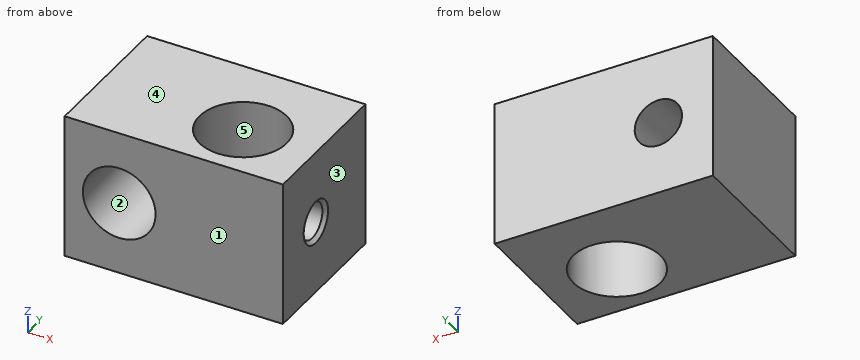
Autodesk Inventor part; units mm, degrees
ref_plane "YZ Plane" through (0, 0, 0) normal (1, 0, 0) x (0, 1, 0)
ref_plane "XZ Plane" through (0, 0, 0) normal (0, 1, 0) x (-1, 0, 0)
ref_plane "XY Plane" through (0, 0, 0) normal (0, 0, 1) x (1, 0, 0)
sketch "Sketch1" plane through (0, 0, 0) normal (0, 0, 1) x (1, 0, 0)
  line L0 (0, 0) -> (30, 0)
  line L1 (30, 0) -> (30, 20)
  line L2 (30, 20) -> (0, 20)
  line L3 (0, 20) -> (0, 0)
  dimension "d0" = 30
  dimension "d1" = 20
extrude "Extrusion1" add sketch "Sketch1" along normal blind 20
sketch "Sketch2" plane through (0, 0, 0) normal (0, -1, 0) x (1, 0, 0)
  line L0 (30, 20) -> (0, 20)
  line L1 (0, 0) -> (0, 20)
  point P0 (7.5, 10)
  dimension "d4" = 7.5
  dimension "d5" = 10
hole "Hole1" at (7.5, 0, 10) direction (0, 1, 0) diameter 6.5 depth 20 tip angle 118 counterbore diameter 10 counterbore depth 13
sketch "Sketch3" plane through (0, 0, 20) normal (0, 0, 1) x (1, 0, 0)
  line L0 (0, 0) -> (0, 20)
  line L1 (0, 20) -> (30, 20)
  point P0 (20, 8)
  dimension "d13" = 20
  dimension "d14" = 12
hole "Hole2" at (20, 8, 20) direction (0, 0, -1) diameter 12 depth 20 tip angle 118
sketch "Sketch4" plane through (30, 0, 0) normal (1, 0, 0) x (0, 0, -1)
  line L0 (0, 0) -> (0, 20)
  line L1 (0, 20) -> (-20, 20)
  point P0 (-10, 8)
  dimension "d22" = 10
  dimension "d23" = 12
hole "Hole3" at (30, 8, 10) direction (-1, 0, 0) diameter 4.917 depth 6 tip angle 118
chamfer "Chamfer1" distance 0.5 angle 45 1 edges at (30, 8, 12.4585)
equation "\"d17\" = d14"
equation "\"d26\" = d14"
properties part number "MANCAL DO EIXO DIANTEIRO(7)" material "Carbon Steel"
Can you work these out from the model? Positions are in its coordinate system, mm. Face numbers are marked on the shaded views. A direction names the side the tool comes from. Coordinates: 2 decimals unless noted, no trailing zeros. Write each loop counter-clockwise with the first axis right and the second up, starting at its lowest first coordinate (ties: lowest second). Pieces come first, ordered by that corner, then holes. Notation, with made-up numbers: (6, -19) -> (10, -19) arc R28 cw to (10, 3) -> close; hole circle Ø6 at (12, -16.5). An arc over 180 degrees is marked (long way). Write each question's results on one line, items separated by ' | '. Start each with the question number.
Q1. Imagine slicing it at A-A (z = 10). Write out the boundary of the cut face in (x, y), then the cut area to 3 significant figures.
Q2. Imagine slicing it at D-D (y = 15.25). Write out the boundary of the cut face in (x, z).
Q3. We'd pull the mould along X, two halves only. Please class the marked faces 3, 4 and 5: +X half, -X half, draft (parallel to the pull), parting line (faces both ways), or undercut.
Q4. Imagine slicing it at B-B (y = 8). Write out the boundary of the cut face in (x, z), then the cut area to 3 significant figures.
Q5. Imagine slicing it at C-C (x = 20). Write out the boundary of the cut face in (y, z).
Q6. On a 3-axis mill with a long thin cutter (end or side, diameter ignored), from which of +Z, -Z, +X, -X, +Y, -Y can I reach the whole of each face in a straight line? I mean the marked faces 1 and 2. Say none if no direction works.
Q7. If I drill on probe 1 along X at (y, z) = (16.25, 10); probe 2 along Y at (x, z) = (20, 5); probe 3 along Z at (x, y) = (7.5, 15.75), over which ranges is the centre line in solid material (lowest first)?
Q8. I'm going to push flat-ended pins straight in: pin 1 (8.5 mm diameter, centred on x = 7.5, z = 10, fed in from -Y); pin 2 (4 mm diameter, centred on y = 8, z = 10, fed in from +X). Where does each tip first touch, or does it pass through?
Taken from the geometry:
1) outline: (0, 0) -> (2.5, 0) -> (2.5, 13) -> (4.25, 13) -> (4.25, 20) -> (0, 20) -> close; (10.75, 13) -> (12.5, 13) -> (12.5, 0) -> (30, 0) -> (30, 5.04) -> (29.5, 5.54) -> (25.47, 5.54) arc R6 cw (long way) to (25.47, 10.46) -> (29.5, 10.46) -> (30, 10.96) -> (30, 20) -> (10.75, 20) -> close | area: 291 mm^2
2) outline: (0, 0) -> (30, 0) -> (30, 20) -> (0, 20) -> close; hole circle Ø6.5 at (7.5, 10)
3) face 3: +X half | face 4: draft | face 5: undercut
4) outline: (0, 0) -> (14, 0) -> (14, 20) -> (0, 20) -> close; (26, 0) -> (30, 0) -> (30, 7.04) -> (29.5, 7.54) -> (26, 7.54) -> close; (26, 12.46) -> (29.5, 12.46) -> (30, 12.96) -> (30, 20) -> (26, 20) -> close; hole circle Ø10 at (7.5, 10) | area: 262 mm^2
5) outline: (0, 0) -> (2, 0) -> (2, 20) -> (0, 20) -> close; (14, 0) -> (20, 0) -> (20, 20) -> (14, 20) -> close
6) face 1: +Z, -Z, +X, -X, -Y | face 2: -Y
7) probe 1: x = 0 to 4.25, 10.75 to 30 | probe 2: y = 0 to 2, 14 to 20 | probe 3: z = 0 to 6.75, 13.25 to 20
8) pin 1: stops at y = 13 | pin 2: stops at x = 14.34
